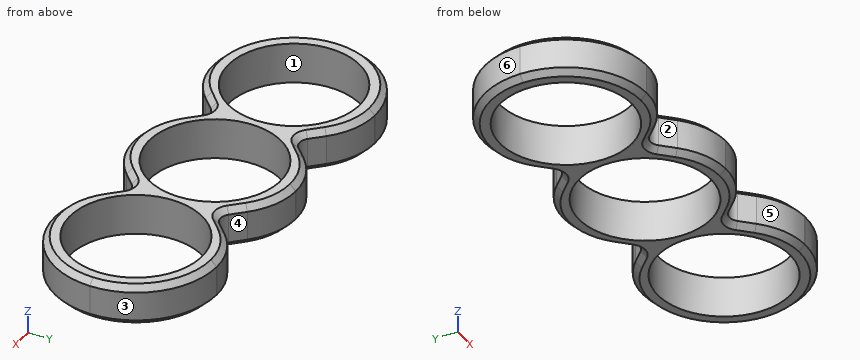
from build123d import *

# Parameters (mm, degrees)
F0_W     = 76
F0_H     = 28
F0_R     = 11.35
F0_R_2   = 11.375
F0_R_3   = 11.4
F1_DEPTH = 7
F3_DEPTH = 7.001
F4_R     = 13.99999
F5_R     = 12
F6_R     = 2
F7_SIZE  = 1


# Not quite as in the source:
# - a fillet or chamfer is up to 0.001 mm smaller than in the source, because OpenCascade refuses the exact size


with BuildPart() as f1:
    # F0 (on Top) → F1 (new body)
    with BuildSketch(Plane.XY):
        Rectangle(F0_W, F0_H)
        with Locations((-24, 0)):
            Circle(F0_R, mode=Mode.SUBTRACT)
        Circle(F0_R_2, mode=Mode.SUBTRACT)
        with Locations((24, 0)):
            Circle(F0_R_3, mode=Mode.SUBTRACT)
    extrude(amount=F1_DEPTH)

    # F2 (on face) → F3 (cut, through all)
    with BuildSketch(Plane.XY.offset(7)):
        Polygon((-5.0125, 14), (-19.0125, 14), (-12.0125, 7), align=None)
        Polygon((18.9875, 14), (4.9875, 14), (11.9875, 7), align=None)
        Polygon((11.9875, -7), (4.9875, -14), (18.9875, -14), align=None)
        Polygon((-5.0125, -14), (-12.0125, -7), (-19.0125, -14), align=None)
    extrude(amount=-F3_DEPTH, mode=Mode.SUBTRACT)

    # F4 (radius 14 in the source; OpenCascade refuses exactly that, so slightly less here)
    f4_edges = [f1.edges().sort_by_distance(p)[0] for p in [
        (-38, -14, 3.5),
        (-38, 14, 3.5),
        (38, -14, 3.5),
        (38, 14, 3.5),
    ]]
    fillet(f4_edges, radius=F4_R)

    # F5
    f5_edges = [f1.edges().sort_by_distance(p)[0] for p in [
        (-19.0125, -14, 3.5),
        (-5.0125, -14, 3.5),
        (4.9875, -14, 3.5),
        (18.9875, -14, 3.5),
        (18.9875, 14, 3.5),
        (4.9875, 14, 3.5),
        (-5.0125, 14, 3.5),
        (-19.0125, 14, 3.5),
    ]]
    fillet(f5_edges, radius=F5_R)

    # F6
    f6_edges = [f1.edges().sort_by_distance(p)[0] for p in [
        (-12.0125, -7, 3.5),
        (11.9875, -7, 3.5),
        (-12.0125, 7, 3.5),
        (11.9875, 7, 3.5),
    ]]
    fillet(f6_edges, radius=F6_R)

    # F7
    f7_edges = [f1.edges().sort_by_distance(p)[0] for p in [
        (-4.634138, -13.086554, 7),
        (-4.634138, -13.086554, 0),
    ]]
    chamfer(f7_edges, length=F7_SIZE)


solid = f1.part
Geometry check sheet. Reference: the model listing, model coordinates, mm. Face numbers are marked on the shaded views. A direction names the side the tool comes from. Round coordinates to 2 decimals unless told otherwise and drop trailing zeros.
Item 1: Gauge pin test, flat ends, axial feed: pin 1 (1 mm diameter, centred on x = 28, z = 5.5, fed in from +Y); pin 2 (1 mm diameter, centred on y = 9, z = 2.5, fed in from -X); pin 3 (1.5 mm diameter, centred on x = -21, z = 2, fed in from -Y); pin 4 (1.5 mm diameter, centred on x = 11, y = -11, fed in from +Z). Record the tip position at first contact, or that the pin passes through.
Item 2: Mould release check, pull along Y, two halves, no side actions. Record for the marked faces 1, 2 and 3: pulls with the +Y half, pulls with the -Y half, needs draft (parallel to the pull), parting line crosses it, or undercut.
Item 3: Cross-section at A-A on z = 4. Count the separate pieces of the cut face and the enclosed holes in it, then the cut area to 3 significant figures.
Item 4: Access from +Z, -Z, +X, -X, +Y, -Y to the whole of each face (thin tool, end or side, straight path). Record for the marked faces 4, 5 and 6.
Item 5: Thickness scan on line 1 (Y direction, x = 0, z = 5) (3 decimals); line 2 (X direction, y = 3.25, z = 5.5); line 3 (X direction, y = -6.5, z = 6.5). Record the ranges inside material, lowest first.
Answer sheet:
1. pin 1: stops at y = 13.56
1. pin 2: stops at x = -35.12
1. pin 3: stops at y = -13.79
1. pin 4: passes through
2. face 1: undercut
2. face 2: pulls with the -Y half
2. face 3: pulls with the +Y half
3. separate pieces: 1
3. enclosed holes: 3
3. area: 523 mm2
4. face 4: +Z, -Z, +Y
4. face 5: +Z, -Z, -Y
4. face 6: +Z, -Z, -X, +Y
5. line 1: y = -14 to -11.375, 11.375 to 14
5. line 2: x = -37.62 to -34.87, -13.13 to -10.9, 10.9 to 13.07, 34.93 to 37.62
5. line 3: x = -35.83 to -33.3, -14.7 to -9.33, 9.33 to 14.63, 33.37 to 35.83
